```python
from build123d import *

# Parameters (mm, degrees)
SKETCH1_R           = 4.111811984
SKETCH1_W           = 4.7
SKETCH1_H           = 3.5
BOSS_EXTRUDE1_DEPTH = 6
CUT_EXTRUDE1_DEPTH  = 6
BOSS_EXTRUDE2_START = 2
SKETCH4_W           = 4.7
SKETCH4_H           = 3.5
BOSS_EXTRUDE2_DEPTH = 2
FILLET1_R           = 1
SKETCH5_W           = 4.7
SKETCH5_H           = 3.5
BOSS_EXTRUDE3_DEPTH = 2


with BuildPart() as part:
    # Sketch1 → Boss-Extrude1 (new body)
    with BuildSketch(Plane(origin=(0, 0, 0), x_dir=(1, 0, 0), z_dir=(0, 1, 0))):
        with Locations(Location((0, 0, 0), (0, 0, 270))):
            Circle(SKETCH1_R)
        Rectangle(SKETCH1_W, SKETCH1_H, mode=Mode.SUBTRACT)
    extrude(amount=BOSS_EXTRUDE1_DEPTH)

    # Sketch3 → Cut-Extrude1 (cut)
    with BuildSketch(Plane(origin=(0, 6, 0), x_dir=(1, 0, 0), z_dir=(0, 1, 0))):
        Polygon((0, -4.111811984), (-6.956919602, 0), (0.821126852, -8.503515518), (6.0147149, -0.720584911), align=None)
    extrude(amount=-CUT_EXTRUDE1_DEPTH, mode=Mode.SUBTRACT)

    # Sketch4 → Boss-Extrude2 (add)
    with BuildSketch(Plane.XZ.offset(BOSS_EXTRUDE2_START)):
        with BuildLine():
            Line((0, 4.111811984), (-3.602153369, 1.982798248))
            ThreePointArc((-3.602153369, 1.982798248), (0.083923032, -4.11095545), (3.518230338, 2.128157202))
            Line((3.518230338, 2.128157202), (0, 4.111811984))
        make_face()
        Rectangle(SKETCH4_W, SKETCH4_H, mode=Mode.SUBTRACT)
    extrude(amount=-BOSS_EXTRUDE2_DEPTH)

    # Fillet1
    # the kernel refuses this fillet: 1 mm, written as the material it takes off along each edge
    with BuildSketch(Plane(origin=(2.152193697, -2, 5.383842759), x_dir=(0, 1, 0), z_dir=(-0.860877478620404, 0, -0.5088123099966979))) as fillet1_piece_1:
        with BuildLine():
            CenterArc((FILLET1_R, FILLET1_R), FILLET1_R, 180, 90)
            Line((0, FILLET1_R), (0, 0))
            Line((0, 0), (FILLET1_R, 0))
        make_face()
    extrude(amount=9.184281107, mode=Mode.SUBTRACT)
    with BuildSketch(Plane(origin=(0, -2, 0), x_dir=(-0.4420339671599803, 0, 0.8969983120813605), z_dir=(0.8969983120813605, 0, 0.4420339671599803))) as fillet1_piece_2:
        with BuildLine():
            CenterArc((4.111811984 - FILLET1_R, -FILLET1_R), FILLET1_R, 0, 90)
            Line((4.111811984 - FILLET1_R, 0), (4.111811984, 0))
            Line((4.111811984, 0), (4.111811984, -FILLET1_R))
        make_face()
    revolve(axis=Axis((0, -2, 0), (0, -1, 0)), revolution_arc=309.871545739, mode=Mode.SUBTRACT)
    with BuildSketch(Plane(origin=(5.695938152, -2, 0.900318175), x_dir=(0, 1, 0), z_dir=(-0.8710831255255876, 0, 0.49113561103281167))) as fillet1_piece_3:
        with BuildLine():
            CenterArc((FILLET1_R, FILLET1_R), FILLET1_R, 180, 90)
            Line((0, FILLET1_R), (0, 0))
            Line((0, 0), (FILLET1_R, 0))
        make_face()
    extrude(amount=9.038914582, mode=Mode.SUBTRACT)

    # Sketch5 → Boss-Extrude3 (add)
    with BuildSketch(Plane.XZ.offset(2)):
        Rectangle(SKETCH5_W, SKETCH5_H)
    extrude(amount=-BOSS_EXTRUDE3_DEPTH)


solid = part.part
```
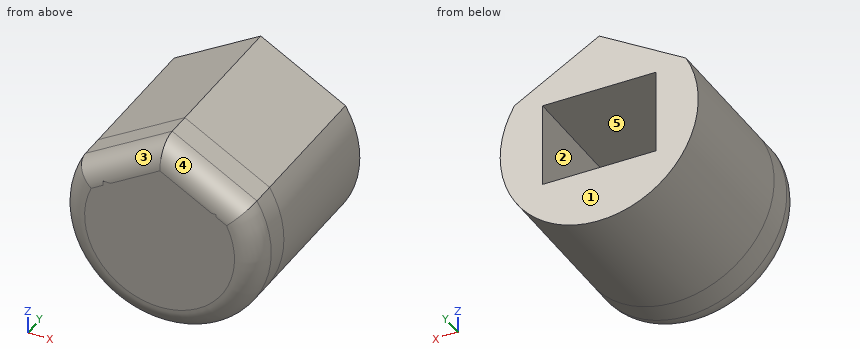
The listing builds one solid part. Answer for the finished solid, in the listing's coordinates (mm). Face numbers are marked on the shaded views. A direction names the side the tool comes from. Coordinates: 2 decimals unless noted, no trailing zeros. Write each loop counter-clockwise with the first axis right and the second up, starting at its lowest first coordinate (ties: lowest second). Pieces come first, ordered by that corner, then holes. Notation, with made-up numbers: (52.25, -29) - (74.25, -29) arc R25 ccw to (74.25, 2) - close; hole circle Ø2 at (70, -15). An arc over 180 degrees is marked (long way). One line per item, written item: value.
1) Find section B-B (z = 0). Give the vertices of the cut face in (x, y).
Geometry check:
outline: (-4.11, -1) arc R1 ccw to (-3.11, -2) - (3.11, -2) arc R1 ccw to (4.11, -1) - (4.11, 6) - (2.35, 6) - (2.35, 0) - (-2.35, 0) - (-2.35, 6) - (-4.11, 6) - close
2) For a pull along Z with two mould halves and no side action, classify the marked faces 1, 2 and 3 as pulls with the +Z half, pulls with the -Z half, needs draft (parallel to the pull), parting line crosses it, or undercut.
Geometry check:
face 1: needs draft
face 2: undercut
face 3: pulls with the +Z half
3) Find section A-A (y = 5.5). Give the vertices of the cut face in (x, z).
Geometry check:
outline: (-3.6, 1.98) arc R4.11 ccw (long way) to (3.52, 2.13) - (0, 4.11) - close; hole (-2.35, -1.75) - (2.35, -1.75) - (2.35, 1.75) - (-2.35, 1.75) - close
4) A tool of negligible diameter and unlimited length cuts with its end or side. For the marked faces 4 and 5, from which of +Z, -Z, +X, -X, +Y, -Y can it reach the whole face along a straight path? Write none if from no direction.
Geometry check:
face 4: +Z, +X, -Y
face 5: +Y
5) Consider line 1 along X through (y, z) = (0.5, 0); line 2 along Z through (x, y) = (-2, 5.25); line 3 along X through (y, z) = (0.75, -0.75). Determine where each line is inside the solid, lowest interval first. Write a range as from..to.
Geometry check:
line 1: x = -4.11..-2.35, 2.35..4.11
line 2: z = -3.59..-1.75, 1.75..2.93
line 3: x = -4.04..-2.35, 2.35..4.04
6) Find section C-C (y = -1.25). Give the vertices of the cut face in (x, z), and give its area (3 significant figures).
Geometry check:
outline: (-3.58, 1.96) arc R4.08 ccw (long way) to (3.5, 2.1) - (0, 4.08) - close
area: 49.2 mm2
